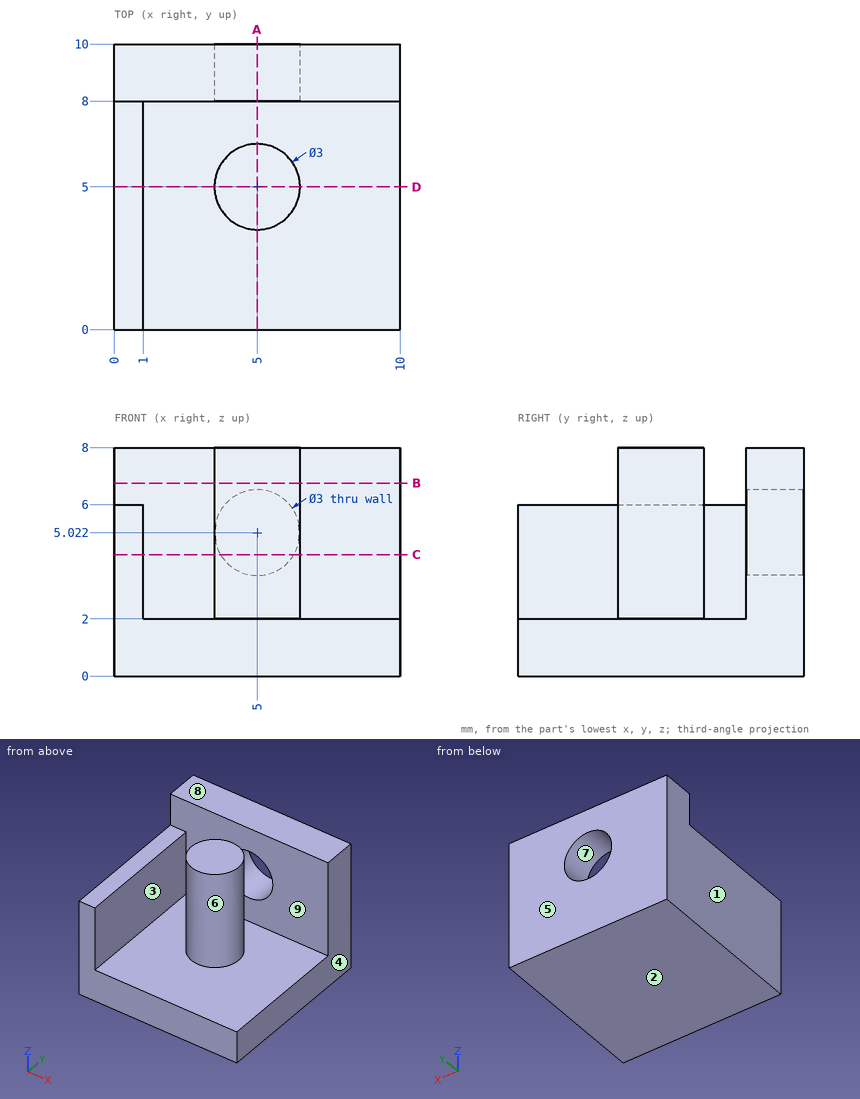
Job drawing, mm, ordinate dimensions from the low corner. One solid piece. A direction names the side the tool comes from. Coordinates: 2 decimals unless noted, no trailing zeros. Order: outer loops, then holes, each group sorted by start corner. A loop starts at its lowest first (then second) coordinate and runs counter-clockwise, first axis right, second up. Notation, with made-up numbers: (38, 0.25) -> (51, 0.25) arc R21 ccw to (51, 35.25) -> close; hole circle Ø2 at (22.25, 76). An arc over 180 degrees is marked (long way). Answer in a Markdown table with one row per item. Add a question column.
Q1. Mould opens along X. For the marked faces 1, 2, 3 and 4 say: +X half, -X half, draft (parallel to the pull), parting line (faces both ways), or undercut.
Q2. Drop flat-ended pins along their axis: pin 1 (6 mm diameter, centred on x = 5, y = 6.5, fed in from -Z); pin 2 (1 mm diameter, centred on x = 2, z = 5.5, fed in from -Y); pin 3 (1.1 mm diameter, centred on x = 0.5, y = 3.5, fed in from +Z); pin 4 (2.5 mm diameter, centred on x = 5, z = 5.02, fed in from -Y). Give the stop position or say it passes through.
Q3. Band-saw the part on B-B, the plane z = 6.75. List the corners of the cut face in (x, y).
Q4. Band-saw the part on A-A, the plane x = 5. List the corners of the cut face in (y, z).
Q5. Which spindle directions (+Z, -Z, +X, -X, +Y, -Y) get a long thin tool onto all of the face, cutting with end or side? Do the marked faces 5, 6, 7, 8 and 9. Say none if no direction does.
Q6. Wall check: line 1 along Z through (x, y) = (5, 8.45); line 2 along Z through (x, y) = (8.75, 0.5); line 3 along Y through (x, z) = (3, 2.5). Give the ranges that are in metal, low to high. Write a range as [from, to].
Q7. Band-saw the part on C-C, the plane z = 4.25. List the corners of the cut face in (x, y).
Q8. Band-saw the part on D-D, the plane y = 5. List the corners of the cut face in (x, z).
Answers follow:
| question | item | result |
|---|---|---|
| 1 | face 1 | -X half |
| 1 | face 2 | draft |
| 1 | face 3 | undercut |
| 1 | face 4 | +X half |
| 2 | pin 1 | z = 0 |
| 2 | pin 2 | y = 8 |
| 2 | pin 3 | z = 6 |
| 2 | pin 4 | y = 3.5 |
| 3 | outline | (0, 8) -> (10, 8) -> (10, 10) -> (0, 10) -> close; circle Ø3 at (5, 5) |
| 4 | outline | (0, 0) -> (10, 0) -> (10, 3.52) -> (8, 3.52) -> (8, 2) -> (6.5, 2) -> (6.5, 8) -> (3.5, 8) -> (3.5, 2) -> (0, 2) -> close; (8, 6.52) -> (10, 6.52) -> (10, 8) -> (8, 8) -> close |
| 5 | face 5 | +Z, -Z, +X, -X, +Y |
| 5 | face 6 | +Z |
| 5 | face 7 | +Y |
| 5 | face 8 | +Z, +X, -X, +Y, -Y |
| 5 | face 9 | +Z, +X |
| 6 | line 1 | [0, 3.52], [6.52, 8] |
| 6 | line 2 | [0, 2] |
| 6 | line 3 | [8, 10] |
| 7 | outline | (0, 0) -> (1, 0) -> (1, 8) -> (3.71, 8) -> (3.71, 10) -> (0, 10) -> close; circle Ø3 at (5, 5); (6.29, 8) -> (10, 8) -> (10, 10) -> (6.29, 10) -> close |
| 8 | outline | (0, 0) -> (10, 0) -> (10, 2) -> (6.5, 2) -> (6.5, 8) -> (3.5, 8) -> (3.5, 2) -> (1, 2) -> (1, 6) -> (0, 6) -> close |
